Verification items for the finished model (mm, model axes). A direction names the side the tool comes from. Give positions to 0.01 mm unless a question says otherwise; leave off trailing zeros. Loops run counter-clockwise (first coordinate to the right, second up) from the corner with the lowest first, then second, coordinate; pieces in that order, holes last. Notation, with made-up numbers: M 25,-34.5 L 64,-34.5 A24 cw 64,3.5 Z; hole C -1.75,73.25 d7. An arc over 180 degrees is marked long. Use a Markdown table: item, result.
Autodesk Inventor part; units mm, degrees
ref_plane "YZ Plane" through (0, 0, 0) normal (1, 0, 0) x (0, 1, 0)
ref_plane "XZ Plane" through (0, 0, 0) normal (0, 1, 0) x (-1, 0, 0)
ref_plane "XY Plane" through (0, 0, 0) normal (0, 0, 1) x (1, 0, 0)
sketch "Эскиз1" plane through (0, 0, 0) normal (0, 1, 0) x (-1, 0, 0)
  circle A0 centre (0, 0) radius 23
  dimension "d0" = 46
extrude "Выдавливание1" add sketch "Эскиз1" along normal blind 25
sketch "Эскиз2" plane through (0, 25, 0) normal (0, 1, 0) x (1, 0, 0)
  circle A0 centre (0, 0) radius 15
  dimension "d3" = 30
extrude "Выдавливание2" add sketch "Эскиз2" along normal blind 35
sketch "Эскиз3" plane through (0, 60, 0) normal (0, 1, 0) x (1, 0, 0)
  line L0 (9, -13) -> (-9, -13)
  line L1 (-9, -13) -> (-9, 13)
  line L2 (-9, 13) -> (9, 13)
  line L3 (9, 13) -> (9, -13)
  line L4 (9, -13) -> (-9, 13) construction
  line L5 (-9, -13) -> (9, 13) construction
  circle A0 centre (0, 0) radius 23
  dimension "d6" = 26
  dimension "d7" = 18
extrude "Выдавливание3" cut sketch "Эскиз3" against normal blind 25
sketch "Эскиз4" plane through (9, 60, 12) normal (1, 0, 0) x (0, 0, -1)
  circle A0 centre (12, -12.5) radius 3.5
  line L0 (0, -25) -> (24, -25)
  point P0 (12, -60)
  dimension "d10" = 7
  dimension "d11" = 12.5
extrude "Выдавливание4" cut sketch "Эскиз4" along normal through all both and the other way through all
sketch "Эскиз5" plane through (0, 0, 0) normal (0, 0, 1) x (1, 0, 0)
  circle A0 centre (0, 12.5) radius 3.5
  point P0 (0, 0)
  dimension "d14" = 7
  dimension "d15" = 12.5
extrude "Выдавливание5" cut sketch "Эскиз5" along normal through all both and the other way through all
properties part number "ДЗ2-1"
(1) Set-up check for faces 1 (the flat face through (9, 45, -3)), 2 (the flat face through (0, 48, -13)), 3 (the flat face through (-9, 45, 3)), 4 (the cylindrical face through (8.06, 34.48, 12.65)), 5 (the flat face through (0, 35, 14)): record each of +Z, -Z, +X, -X, +Y, -Y from which the full face is reachable in a straight line by a thin tool's end or side.
Results below:
| item | result |
|---|---|
| face 1 | +Z, -Z, +X, +Y |
| face 2 | -Z, +X, -X, +Y |
| face 3 | +Z, -Z, -X, +Y |
| face 4 | +Y |
| face 5 | +Z, +X, -X, +Y |
(2) Gauge pin test, flat ends, axial feed: P1, Ø5, axis at y = 30.5, z = 14.5, coming from the -X side; P2, Ø10, axis at x = -1.5, z = -15.5, coming from the +Y side; P3, Ø12, axis at x = 2.5, y = 45.5, coming from the +Z side; P4, Ø3, axis at x = 12.5, z = 3, coming from the +Y side. Record the tip position at first contact, or that the pin passes through.
Results below:
| item | result |
|---|---|
| P1 | x = -9 |
| P2 | y = 60 |
| P3 | z = 13 |
| P4 | y = 35 |
(3) Cross-section at D-D on x = 6.5. Record the cut outline in (y, z), then the cut area to 3 significant figures.
Results below:
| item | result |
|---|---|
| outline | M 0,-22.06 L 25,-22.06 L 25,-13.52 L 35,-13.52 L 35,-13 L 60,-13 L 60,13 L 35,13 L 35,13.52 L 25,13.52 L 25,22.06 L 0,22.06 Z; hole C 47.5,0 d7 |
| area | 1,990 mm^2 |
(4) Cross-section at B-B on x = 0. Record the cut outline in (y, z).
Results below:
| item | result |
|---|---|
| outline | M 0,-23 L 9,-23 L 9,23 L 0,23 Z; M 16,-23 L 25,-23 L 25,-15 L 35,-15 L 35,-13 L 60,-13 L 60,13 L 35,13 L 35,15 L 25,15 L 25,23 L 16,23 Z; hole C 47.5,0 d7 |
(5) Cross-section at C-C on z = 0. Record the cut outline in (x, y), then the cut area to 3 significant figures.
Results below:
| item | result |
|---|---|
| outline | M -23,0 L 23,0 L 23,25 L 15,25 L 15,35 L 9,35 L 9,44 L -9,44 L -9,35 L -15,35 L -15,25 L -23,25 Z; M -9,51 L 9,51 L 9,60 L -9,60 Z; hole C 0,12.5 d7 |
| area | 1,740 mm^2 |
(6) Cross-section at A-A on y = 47.5. Record the cut outline in (x, z), then the cut area to 3 significant figures.
Results below:
| item | result |
|---|---|
| outline | M -9,-12 A15 ccw -7.48,-13 L 7.48,-13 A15 ccw 9,-12 L 9,-3.5 L -9,-3.5 Z; M -9,3.5 L 9,3.5 L 9,12 A15 ccw 7.48,13 L -7.48,13 A15 ccw -9,12 Z |
| area | 339 mm^2 |
(7) Draft check along Y on faces 6 (the flat face through (0, 48, 13)), 7 (the cylindrical face through (0, 51, 0)), 8 (the flat face through (11, 35, 0)). Enter one of: +Y half, -Y half, draft (parallel to the pull), parting line (faces both ways), or undercut.
Results below:
| item | result |
|---|---|
| face 6 | draft |
| face 7 | undercut |
| face 8 | +Y half |
(8) Material ranges on line 1 (Y direction, x = 5.25, z = 0); line 2 (Y direction, x = 0, z = -6); line 3 (Y direction, x = 1.75, z = 0), recorded low to high.
Results below:
| item | result |
|---|---|
| line 1 | 0 to 44, 51 to 60 |
| line 2 | 0 to 9, 16 to 60 |
| line 3 | 0 to 9.47, 15.53 to 44, 51 to 60 |
